Build history of the part. All positions in model axes, mm. A direction names the side the tool comes from. Round coordinates to 2 decimals unless told otherwise and drop trailing zeros. Loops run counter-clockwise (first coordinate to the right, second up) from the corner with the lowest first, then second, coordinate; pieces in that order, holes last. Notation, with made-up numbers: (51.5, 36.5) - (93.5, 36.5) arc R20 cw to (93.5, 49.5) - close; hole circle Ø9 at (51.25, 63.25). An arc over 180 degrees is marked (long way). Use one line per item in the form item = value. Start each with the question number.
Q1. Pin check, flat tips, straight feed: pin 1 (5 mm diameter, centred on x = -2, z = 21, fed in from +Y); pin 2 (2.5 mm diameter, centred on x = -30.91, y = -8.28, fed in from +Z); pin 3 (1.5 mm diameter, centred on y = 25, z = 7.5, fed in from -X). Stop position of each tip, or through.
Q2. Saw through at A-A (z = 14.5). Give the cut face in (x, y).
Q3. Mould opens along X. For faces 3 (the face through (-33.727, -25.861, 4.479)), 4 (the face through (-29.002, -7.681, 25.605)), 5 (the face through (-26.9, -33.1, 3)) say: released by +X, released by -X, zero draft, split by the parting line, or undercut.
Q4. 3-axis set-ups, long thin cutter, end or side, ignore diameter. For faces 1 (the face through (-4.88, 37.18, 4.97)), 2 (the face through (-26, 17, 2)): which of +Z, -Z, +X, -X, +Y, -Y reach the whole face in a straight line?
Q5. Saw through at B-B (z = 28.5). Give the cut face in (x, y), then the cut area to 3 significant figures.
Q6. Drill centre lines: line 1 (Y direction, x = 3.5, z = 5); line 2 (Y direction, x = 7, z = 6); line 3 (Z direction, x = 19, y = -13). Where is each one in solid material? Low to high.
```python
from build123d import *

# Parameters (mm, degrees)
SKETCH1_R           = 45
BOSS_EXTRUDE1_DEPTH = 3
SKETCH2_R           = 42.5
SKETCH2_R_2         = 37.5
BOSS_EXTRUDE2_DEPTH = 4
CHAMFER1_SIZE       = 2
FILLET1_R           = 1
BOSS_EXTRUDE3_DEPTH = 30
SKETCH4_R           = 2
CUT_EXTRUDE1_DEPTH  = 15
CIRPATTERN1_COUNT   = 2
SKETCH5_R           = 1.75
CUT_EXTRUDE2_DEPTH  = 4


with BuildPart() as part:
    # Sketch1 → Boss-Extrude1 (new body)
    with BuildSketch(Plane.XY):
        Circle(SKETCH1_R)
    extrude(amount=BOSS_EXTRUDE1_DEPTH)

    # Sketch2 → Boss-Extrude2 (add)
    with BuildSketch(Plane.XY.offset(3)):
        Circle(SKETCH2_R)
        Circle(SKETCH2_R_2, mode=Mode.SUBTRACT)
    extrude(amount=BOSS_EXTRUDE2_DEPTH)

    # Chamfer1
    chamfer1_edges = [part.edges().sort_by_distance(p)[0] for p in [
        (-45, 0, 0),
    ]]
    chamfer(chamfer1_edges, length=CHAMFER1_SIZE)

    # Fillet1
    fillet1_edges = [part.edges().sort_by_distance(p)[0] for p in [
        (-42.5, 0, 7),
    ]]
    fillet(fillet1_edges, radius=FILLET1_R)

    # Sketch3 → Boss-Extrude3 (add)
    with BuildSketch(Plane.XY.offset(3)):
        with BuildLine():
            Line((-36, 0), (-28, 0))
            ThreePointArc((-28, 0), (-19.798989873, -19.798989873), (0, -28))
            Line((0, -28), (0, -36))
            ThreePointArc((0, -36), (-25.455844123, -25.455844123), (-36, 0))
        make_face()
    boss_extrude3 = extrude(amount=BOSS_EXTRUDE3_DEPTH)

    # Sketch4 → Cut-Extrude1 (cut)
    with BuildSketch(Plane.XY.offset(33)):
        with Locations((-30.909626441, -8.282209443)):
            Circle(SKETCH4_R)
        with Locations((-8.282209443, -30.909626441)):
            Circle(SKETCH4_R)
    cut_extrude1 = extrude(amount=-CUT_EXTRUDE1_DEPTH, mode=Mode.SUBTRACT)

    # CirPattern1: Boss-Extrude3, Cut-Extrude1 ×2 about axis
    cirpattern1_axis = Axis((0, 0, 0), (0, 0, 1))
    for i in range(1, CIRPATTERN1_COUNT):
        add(boss_extrude3.rotate(cirpattern1_axis, i * 360 / CIRPATTERN1_COUNT))
        add(cut_extrude1.rotate(cirpattern1_axis, i * 360 / CIRPATTERN1_COUNT), mode=Mode.SUBTRACT)

    # Sketch5 → Cut-Extrude2 (cut, through all)
    with BuildSketch(Plane.XY.offset(3)):
        with Locations((-25.809397513, 18.738329701)):
            Circle(SKETCH5_R)
        with Locations((-13.788582233, 6.717514421)):
            Circle(SKETCH5_R)
    extrude(amount=-CUT_EXTRUDE2_DEPTH, mode=Mode.SUBTRACT)


solid = part.part
```
Report:
q1.pin_1 = 36
q1.pin_2 = 18
q1.pin_3 = -34.07
q2.outline = (-36, 0) arc R36 ccw to (0, -36) - (0, -28) arc R28 cw to (-28, 0) - close; (0, 28) arc R28 cw to (28, 0) - (36, 0) arc R36 ccw to (0, 36) - close
q3.face_3 = split by the parting line
q3.face_4 = undercut
q3.face_5 = zero draft
q4.face_1 = +Z
q4.face_2 = +Z, -Z
q5.outline = (-36, 0) arc R36 ccw to (0, -36) - (0, -28) arc R28 cw to (-28, 0) - close; (0, 28) arc R28 cw to (28, 0) - (36, 0) arc R36 ccw to (0, 36) - close; hole circle Ø4 at (-30.91, -8.28); hole circle Ø4 at (-8.28, -30.91); hole circle Ø4 at (8.28, 30.91); hole circle Ø4 at (30.91, 8.28)
q5.area = 754 mm²
q6.line_1 = -42.36 to -37.34, 27.78 to 35.83, 37.34 to 42.36
q6.line_2 = -41.92 to -36.84, 27.11 to 35.31, 36.84 to 41.92
q6.line_3 = 0 to 3
